The drawing under review shows one solid part. Ordinate dimensions are in mm from its lowest x, y, z. Round coordinates to 2 decimals unless told otherwise and drop trailing zeros. Order: outer loops, then holes, each group sorted by start corner. A loop starts at its lowest first (then second) coordinate and runs counter-clockwise, first axis right, second up. Notation, with made-up numbers: (81, 27.5) -> (86, 27.5) arc R31 ccw to (86, 66.5) -> close; hole circle Ø2 at (27, -13.75). An arc over 180 degrees is marked (long way). Use a Markdown table: item, result. Add a question column.
1) Clearance check with flat-ended pins moving along their axes: P1, Ø3.5, axis at x = 105, z = 17.5, coming from the +Y side; P2, Ø1.5, axis at x = 74.5, z = 114.5, coming from the -Y side. State where each tip first meets the part, or that it passes through.
2) Draft analysis for pull direction Y (two halves, no side actions). For the marked faces 1 and 2, state which applies: pulls with the +Y half, pulls with the -Y half, needs draft (parallel to the pull), parting line crosses it, or undercut.
3) Wall thickness on line 1 along X through (y, z) = (2.9, 17.5); line 2 along Z through (x, y) = (104, 2.4); line 3 along Z through (x, y) = (102.5, 4.2): over which ranges is each line inside the solid? List them lowest first. Write a range as [from, to].
4) Consider section B-B (x = 105). State the section outline as (y, z) points, plus the area to 3 significant figures.
5) Consider section A-A (z = 112.5). State the section outline as (x, y) points, plus the area to 3 significant figures.
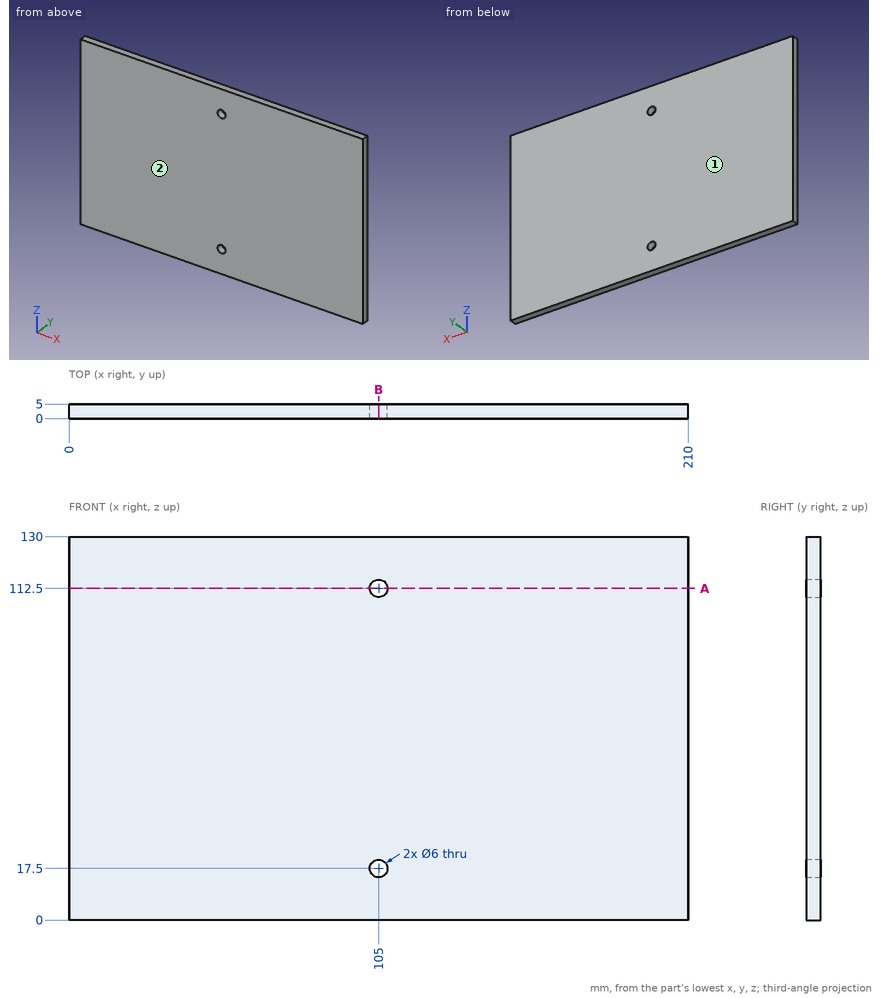
Results list:
| question | item | result |
|---|---|---|
| 1 | P1 | through |
| 1 | P2 | y = 0 |
| 2 | face 1 | pulls with the +Y half |
| 2 | face 2 | pulls with the -Y half |
| 3 | line 1 | [0, 102], [108, 210] |
| 3 | line 2 | [0, 14.67], [20.33, 109.67], [115.33, 130] |
| 3 | line 3 | [0, 15.84], [19.16, 110.84], [114.16, 130] |
| 4 | outline | (0, 0) -> (5, 0) -> (5, 14.5) -> (0, 14.5) -> close; (0, 20.5) -> (5, 20.5) -> (5, 109.5) -> (0, 109.5) -> close; (0, 115.5) -> (5, 115.5) -> (5, 130) -> (0, 130) -> close |
| 4 | area | 590 mm2 |
| 5 | outline | (0, 0) -> (102, 0) -> (102, 5) -> (0, 5) -> close; (108, 0) -> (210, 0) -> (210, 5) -> (108, 5) -> close |
| 5 | area | 1,020 mm2 |
